The model under review builds one solid part; all positions refer to its coordinate system, in mm. A direction names the side the tool comes from. Round coordinates to 2 decimals unless told otherwise and drop trailing zeros. Order: outer loops, then holes, each group sorted by start corner. A loop starts at its lowest first (then second) coordinate and runs counter-clockwise, first axis right, second up.
1) Consider section C-C (x = 25.5). Give the boundary of the cut face in (y, z).
2) Consider section A-A (x = 39.5). Give the boundary of the cut face in (y, z), then the cut area to 3 significant figures.
3) Clearance check with flat-ended pins moving along their axes: P1, Ø12, axis at y = 19, z = 57.5, coming from the -X side; P2, Ø6, axis at y = -18, z = 10, coming from the +X side; P3, Ø13.5, axis at y = -2.5, z = 48, coming from the -X side. State where each tip first meets the part, or that it passes through.
4) Mouldability with a two-part tool opening along X and no side actions: class faces 4 (the face through (15.508, 22.579, 39.514)), 5 (the face through (37.64, -37.78, 39.51)), 6 (the face through (88.43, -14.91, 39.51)) as pulls with the +X half, pulls with the -X half, needs draft (parallel to the pull), parting line crosses it, or undercut.
5) Machinability: for faces 1 (the face through (69.95, 34.38, 39.51)), 2 (the face through (17.868, -25.826, 39.514)), 3 (the face through (88.43, 14.91, 39.51)), which of the approach directions +Z, -Z, +X, -X, +Y, -Y give a long, thin tool a straight path to every point of the face, cutting with its end or side? Answer none if there is none.
6) Consider section B-B (x = 57). Give the boundary of the cut face in (y, z).
7) To check wall thickness, follow L1, parallel to Y at x = 15.5, z = 26.5; L2, parallel to Y at x = 79.5, z = 56.5; L3, parallel to X at y = 3, z = 18.5. State the ranges of each line that lie inside material, in increasing order.
from build123d import *

# Parameters (mm, degrees)
SKETCH008_R           = 39.75
PAD007_DEPTH          = 80.15
PAD008_DEPTH          = 80.15
POLARPATTERN005_COUNT = 15
POCKET008_DEPTH       = 80.151


with BuildPart() as part:
    # Sketch008 → Pad007 (new body)
    with BuildSketch(Plane.XY):
        Circle(SKETCH008_R)
    extrude(amount=PAD007_DEPTH)

    # Sketch006 → Pad008 (join)
    with BuildSketch(Plane.XY):
        with BuildLine():
            ThreePointArc((42.723676, -1.5), (42.75, 0), (42.723676, 1.5))
            Line((39.671306, 2.5), (42.723676, 1.5))
            Line((39.671306, 2.5), (26.5, 0))
            Line((26.5, 0), (39.671306, -2.5))
            Line((39.671306, -2.5), (42.723676, -1.5))
        make_face()
    pad008 = extrude(amount=PAD008_DEPTH)

    # PolarPattern005: Pad008 ×15 about axis
    polarpattern005_axis = Axis((0, 0, 0), (0, 0, 1))
    for i in range(1, POLARPATTERN005_COUNT):
        add(pad008.rotate(polarpattern005_axis, i * 360 / POLARPATTERN005_COUNT))

    # Sketch007 → Pocket008 (cut, through all)
    with BuildSketch(Plane.XY):
        Polygon((14.3875, 8.306627), (0, 16.613254), (-14.3875, 8.306627), (-14.3875, -8.306627), (0, -16.613254), (14.3875, -8.306627), align=None)
    extrude(amount=POCKET008_DEPTH, mode=Mode.SUBTRACT)


with BuildPart() as part_1:
    # Body011 placement: moved
    add(part.part.moved(Location((50, 0, 0))))


solid = part_1.part
Answer below:
1. outline: (-31.3, 0) - (31.3, 0) - (31.3, 80.15) - (-31.3, 80.15) - close
2. outline: (-38.34, 0) - (-10.55, 0) - (-10.55, 80.15) - (-38.34, 80.15) - close; (10.55, 0) - (38.34, 0) - (38.34, 80.15) - (10.55, 80.15) - close
2. area: 4,450 mm2
3. P1: stops at x = 12.44
3. P2: stops at x = 89.64
3. P3: stops at x = 7.9
4. face 4: pulls with the -X half
4. face 5: undercut
4. face 6: pulls with the +X half
5. face 1: +Z, -Z, +Y
5. face 2: +Z, -Z, -Y
5. face 3: +Z, -Z, +X
6. outline: (-39.13, 0) - (-12.57, 0) - (-12.57, 80.15) - (-39.13, 80.15) - close; (12.57, 0) - (39.13, 0) - (39.13, 80.15) - (12.57, 80.15) - close
7. L1: y = -25.25 to -22.59, -19.74 to 19.74, 22.59 to 25.25
7. L2: y = -30.94 to -30.29, -26.64 to 26.64, 30.29 to 30.94
7. L3: x = 10.36 to 35.61, 64.39 to 89.64
